Model file for the job. Use its own axes, mm. A direction names the side the tool comes from. Give positions to 0.01 mm unless a question says otherwise; leave off trailing zeros. Loops run counter-clockwise (first coordinate to the right, second up) from the corner with the lowest first, then second, coordinate; pieces in that order, holes last. Notation, with made-up numbers: M 64.5,68.5 L 81.5,68.5 A24 cw 81.5,101.5 Z; hole C 51.5,77.5 d11. An arc over 180 degrees is marked long. Answer in a Markdown table with one row per item.
```python
from build123d import *

# Parameters (mm, degrees)
F3_DEPTH = 50
F5_DEPTH = 50


with BuildPart() as f1:
    # F0 (on Top) → F1 (revolve)
    with BuildSketch(Plane.XY):
        Polygon((-300, 5), (-300, 0), (-100, 0), (-50, 0), (50, 0), (100, 0), (300, 0), (300, 5), align=None)
        Polygon((-50, 0), (-100, 0), (-100, -25), (-90, -25), (-90, -15), (-60, -15), (-60, -25), (-50, -25), align=None)
        Polygon((100, 0), (50, 0), (50, -25), (60, -25), (60, -15), (90, -15), (90, -25), (100, -25), align=None)
    revolve(axis=Axis((0, 5, 0), (1, 0, 0)))

    # F2 (on face) → F3 (join)
    with BuildSketch(Plane(origin=(-300, 0, 0), x_dir=(0, -1, 0), z_dir=(-1, 0, 0))):
        with BuildLine():
            Line((0, -5.2596899241), (0, 0))
            ThreePointArc((0, 0), (-0.527864045, -2.2360679775), (-2, -4))
            Line((-2, -4), (-2, -5.2596899241))
            Line((-2, -5.2596899241), (0, -5.2596899241))
        make_face()
        with BuildLine():
            ThreePointArc((0, 0), (-0.527864045, 2.2360679775), (-2, 4))
            Line((-2, 4), (-2, -4))
            ThreePointArc((-2, -4), (-0.527864045, -2.2360679775), (0, 0))
        make_face()
        with BuildLine():
            Line((0, 4.7403100759), (-2, 4.7403100759))
            Line((-2, 4.7403100759), (-2, 4))
            ThreePointArc((-2, 4), (-0.527864045, 2.2360679775), (0, 0))
            Line((0, 0), (0, 4.7403100759))
        make_face()
    extrude(amount=F3_DEPTH)

    # F4 (on face) → F5 (join)
    with BuildSketch(Plane.YZ.offset(300)):
        with BuildLine():
            ThreePointArc((2, -4), (0.527864045, -2.2360679775), (0, 0))
            Line((0, 0), (0, -5))
            Line((0, -5), (2, -5))
            Line((2, -5), (2, -4))
        make_face()
        with BuildLine():
            Line((2, 5), (0, 5))
            Line((0, 5), (0, 0))
            ThreePointArc((0, 0), (0.527864045, 2.2360679775), (2, 4))
            Line((2, 4), (2, 5))
        make_face()
        with BuildLine():
            ThreePointArc((2, 4), (0.527864045, 2.2360679775), (0, 0))
            ThreePointArc((0, 0), (0.527864045, -2.2360679775), (2, -4))
            Line((2, -4), (2, 4))
        make_face()
    extrude(amount=F5_DEPTH)


solid = f1.part
```
Q1. Probe probe 1 along X at (y, z) = (26, -15); probe 2 along X at (y, z) = (-1.5, -11.5); probe 3 along Z at (x, y) = (71, 7). List the from-to ranges inside material, lowest first.
Reported:
| item | result |
|---|---|
| probe 1 | -100 to -90, -60 to -50, 50 to 60, 90 to 100 |
| probe 2 | -100 to -50, 50 to 100 |
| probe 3 | -19.9 to 19.9 |
Q2. 3-axis set-ups, long thin cutter, end or side, ignore diameter. For faces 1 (the face through (90, 11, 20)), 2 (the face through (-94.93, -23.615, -9.011)): which of +Z, -Z, +X, -X, +Y, -Y reach the whole face in a straight line?
Reported:
| item | result |
|---|---|
| face 1 | none |
| face 2 | +X, -X |
Q3. Mould opens along X. For faces 3 (the face through (50, 5, 6)), 4 (the face through (-54.93, -23.615, -9.011)) say: released by +X, released by -X, zero draft, split by the parting line, or undercut.
Reported:
| item | result |
|---|---|
| face 3 | undercut |
| face 4 | zero draft |
Q4. Drop flat-ended pins along their axis: pin 1 (18 mm diameter, centred on y = 8.5, z = -9, fed in from -X); pin 2 (5 mm diameter, centred on y = 25.5, z = 7.5, fed in from +X); pin 3 (8 mm diameter, centred on x = -2, z = -4, fed in from -Y); pin 4 (3 mm diameter, centred on x = 323, z = 1, fed in from +Y). Give the stop position or say it passes through.
Reported:
| item | result |
|---|---|
| pin 1 | x = -350 |
| pin 2 | x = 100 |
| pin 3 | y = 0 |
| pin 4 | y = 2 |
Q5. Saw through at A-A (x = 192). Give the cut face in (y, z).
Reported:
| item | result |
|---|---|
| outline | C 5,0 d10 |
